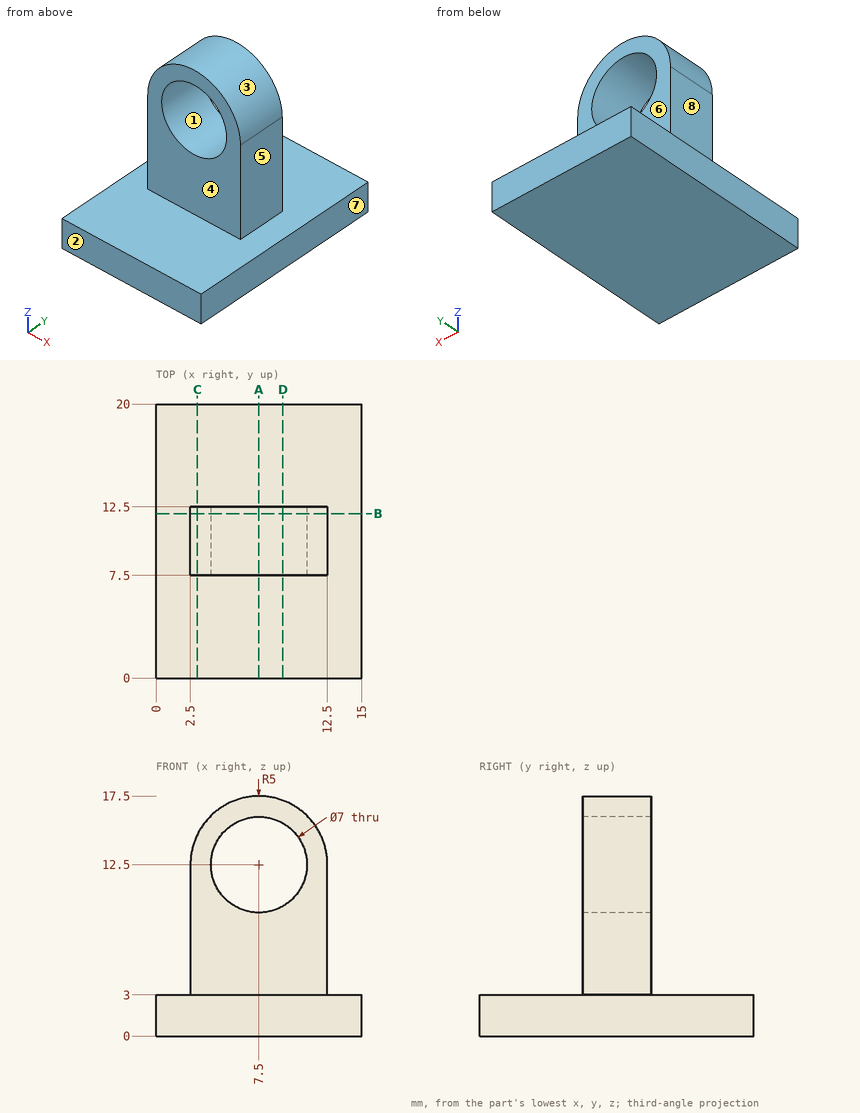
Design review of the part shown in the three views and the two pictorial views. Dimensions are in mm from the part's minimum x, y and z. A direction names the side the tool comes from. Coordinates: 2 decimals unless noted, no trailing zeros. Write each loop counter-clockwise with the first axis right and the second up, starting at its lowest first coordinate (ties: lowest second). Pieces come first, ordered by that corner, then holes.
1) The part is to be moulded in two halves that separate along X. For the marked faces 1, 2 and 3, say which applies: pulls with the +X half, pulls with the -X half, needs draft (parallel to the pull), parting line crosses it, or undercut.
2) Machinability: for the marked faces 4, 5, 6, 7 and 8, which of the approach directions +Z, -Z, +X, -X, +Y, -Y give a long, thin tool a straight path to every point of the face, cutting with its end or side? Answer none if there is none.
3) We need section D-D on x = 9.25. State the section outline as (y, z) points, then the cut area to 3 significant figures.
4) We need section A-A on x = 7.5. State the section outline as (y, z) points, then the cut area to 3 significant figures.
5) Clearance check with flat-ended pins moving along their axes: pin 1 Ø3 at (x, y) = (13, 9) entering from +Z; pin 2 Ø2.5 at (y, z) = (10, 7.5) entering from -X; pin 3 Ø5.5 at (y, z) = (10.5, 8) entering from +X; pin 4 Ø5.5 at (x, z) = (7.5, 12.5) entering from -Y. State where each tip first meets the part, or that it passes through.
6) We need section B-B on y = 12. State the section outline as (x, z) points.
7) To check wall thickness, follow probe 1 along X at (y, z) = (8.75, 12.5); probe 2 along Z at (x, y) = (10.5, 2); probe 3 along Y at (x, z) = (10, 4). State the ranges of each line that lie inside material, in increasing order.
8) We need section C-C on x = 3. State the section outline as (y, z) points, then the cut area to 3 significant figures.
Answer list:
1. face 1: undercut
1. face 2: needs draft
1. face 3: parting line crosses it
2. face 4: +Z, +X, -X, -Y
2. face 5: +Z, +X, +Y, -Y
2. face 6: +Z, +X, -X, +Y
2. face 7: +Z, -Z, +X, +Y, -Y
2. face 8: +Z, -X, +Y, -Y
3. outline: (0, 0) - (20, 0) - (20, 3) - (12.5, 3) - (12.5, 9.47) - (7.5, 9.47) - (7.5, 3) - (0, 3) - close; (7.5, 15.53) - (12.5, 15.53) - (12.5, 17.18) - (7.5, 17.18) - close
3. area: 101 mm2
4. outline: (0, 0) - (20, 0) - (20, 3) - (12.5, 3) - (12.5, 9) - (7.5, 9) - (7.5, 3) - (0, 3) - close; (7.5, 16) - (12.5, 16) - (12.5, 17.5) - (7.5, 17.5) - close
4. area: 97.5 mm2
5. pin 1: stops at z = 15.5
5. pin 2: stops at x = 2.5
5. pin 3: stops at x = 12.5
5. pin 4: passes through
6. outline: (0, 0) - (15, 0) - (15, 3) - (12.5, 3) - (12.5, 12.5) arc R5 ccw to (2.5, 12.5) - (2.5, 3) - (0, 3) - close; hole circle Ø7 at (7.5, 12.5)
7. probe 1: x = 2.5 to 4, 11 to 12.5
7. probe 2: z = 0 to 3
7. probe 3: y = 7.5 to 12.5
8. outline: (0, 0) - (20, 0) - (20, 3) - (12.5, 3) - (12.5, 14.68) - (7.5, 14.68) - (7.5, 3) - (0, 3) - close
8. area: 118 mm2
